Check sheet for the modelled part. Datum: model origin and axes. Units: mm. A direction names the side the tool comes from. Give positions to 0.01 mm unless a question says otherwise; leave off trailing zeros. Order: outer loops, then holes, each group sorted by start corner. A loop starts at its lowest first (then second) coordinate and runs counter-clockwise, first axis right, second up. Notation, with made-up numbers: M -14,78 L 11,78 A30 ccw 11,103 Z; hole C 47.5,-21 d8. An arc over 180 degrees is marked long. Answer in a Markdown table with one row per item. Add a question column.
from build123d import *

# Parameters (mm, degrees)
SKETCH_W           = 180
SKETCH_H           = 180
SKETCH_R           = 2.5
PAD_DEPTH          = 80
SKETCH001_W        = 120
SKETCH001_H        = 80
POCKET_DEPTH       = 11
POCKET002_DEPTH    = 70
POLARPATTERN_COUNT = 4
POCKET003_DEPTH    = 10
SKETCH005_W        = 10
SKETCH005_H        = 30
SKETCH005_H_2      = 25
POCKET004_DEPTH    = 70
SKETCH002_R        = 3
POCKET007_DEPTH    = 11


with BuildPart() as part:
    # Sketch (on Sketch) → Pad (new body)
    with BuildSketch(Plane.XY):
        Rectangle(SKETCH_W, SKETCH_H)
        with Locations((-84, 84)):
            Circle(SKETCH_R, mode=Mode.SUBTRACT)
        with Locations((84, 84)):
            Circle(SKETCH_R, mode=Mode.SUBTRACT)
        with Locations((84, -84)):
            Circle(SKETCH_R, mode=Mode.SUBTRACT)
        with Locations((-84, -84)):
            Circle(SKETCH_R, mode=Mode.SUBTRACT)
        with Locations((-85, 55)):
            Circle(SKETCH_R, mode=Mode.SUBTRACT)
        with Locations((-85, -55)):
            Circle(SKETCH_R, mode=Mode.SUBTRACT)
        with Locations((85, -55)):
            Circle(SKETCH_R, mode=Mode.SUBTRACT)
        with Locations((85, 55)):
            Circle(SKETCH_R, mode=Mode.SUBTRACT)
        with BuildLine():
            Line((-70, 80), (70, 80))
            ThreePointArc((80, 70), (77.071068, 77.071068), (70, 80))
            Line((80, 70), (80, 63.660254))
            ThreePointArc((80, 63.660254), (75, 55), (80, 46.339746))
            Line((80, 46.339746), (80, -46.339746))
            ThreePointArc((80, -46.339746), (75, -55), (80, -63.660254))
            Line((80, -63.660254), (80.000001, -70))
            ThreePointArc((70.000001, -80), (77.071069, -77.071068), (80.000001, -70))
            Line((70.000001, -80), (-69.999999, -80))
            ThreePointArc((-79.999999, -70), (-77.071066, -77.071068), (-69.999999, -80))
            Line((-79.999999, -70), (-79.999999, -63.660253))
            ThreePointArc((-79.999999, -63.660253), (-75, -55), (-79.999999, -46.339747))
            Line((-79.999999, -46.339747), (-79.999999, 46.339747))
            ThreePointArc((-79.999999, 46.339747), (-75, 55), (-79.999999, 63.660253))
            Line((-79.999999, 63.660253), (-79.999999, 69.994765))
            ThreePointArc((-70, 80), (-77.072918, 77.069217), (-79.999999, 69.994765))
        make_face(mode=Mode.SUBTRACT)
    extrude(amount=PAD_DEPTH)

    # Sketch001 (on Face1 of Pad) → Pocket (cut)
    with BuildSketch(Plane(origin=(0, 90, 0), x_dir=(-1, 0, 0), z_dir=(0, 1, 0))):
        with Locations((0, 40)):
            Rectangle(SKETCH001_W, SKETCH001_H)
    extrude(amount=-POCKET_DEPTH, mode=Mode.SUBTRACT)

    # Sketch003 → Pocket002 (cut)
    with BuildSketch(Plane.XY.offset(80)):
        Polygon((-90, 90), (-70, 90), (-90, 70), align=None)
    pocket002 = extrude(amount=-POCKET002_DEPTH, mode=Mode.SUBTRACT)

    # PolarPattern: Pocket002 ×4 about axis
    polarpattern_axis = Axis((0, 0, 80), (0, 0, 1))
    for i in range(1, POLARPATTERN_COUNT):
        add(pocket002.rotate(polarpattern_axis, i * 360 / POLARPATTERN_COUNT), mode=Mode.SUBTRACT)

    # Sketch004 (on Face2 of PolarPattern) → Pocket003 (cut)
    with BuildSketch(Plane(origin=(0, 0, 0), x_dir=(1, 0, 0), z_dir=(0, 0, -1))):
        Polygon((-90, 60), (-83.5, 60), (-80, 57), (-80, 53), (-83.5, 50), (-90, 50), align=None)
        Polygon((83.5, 60), (90, 60), (90, 50), (83.5, 50), (80, 53), (80, 57), align=None)
        Polygon((83.5, -50), (90, -50), (90, -60), (83.5, -60), (80, -57), (80, -53), align=None)
        Polygon((-90, -50), (-83.5, -50), (-80, -53), (-80, -57), (-83.5, -60), (-90, -60), align=None)
    extrude(amount=-POCKET003_DEPTH, mode=Mode.SUBTRACT)

    # Sketch005 (on Face6 of Pocket003) → Pocket004 (cut)
    with BuildSketch(Plane.XY.offset(10)):
        with Locations((-75, 55)):
            Rectangle(SKETCH005_W, SKETCH005_H)
        with Locations((75, 55)):
            Rectangle(SKETCH005_W, SKETCH005_H)
        with Locations((75, -55)):
            Rectangle(SKETCH005_W, SKETCH005_H)
        with Locations((-75, -52.5)):
            Rectangle(SKETCH005_W, SKETCH005_H_2)
    extrude(amount=POCKET004_DEPTH, mode=Mode.SUBTRACT)

    # Sketch002 (on Face30 of Pocket004) → Pocket007 (cut)
    with BuildSketch(Plane(origin=(0, -80, 0), x_dir=(-1, 0, 0), z_dir=(0, 1, 0))):
        with Locations((-50, 5)):
            Circle(SKETCH002_R)
    extrude(amount=-POCKET007_DEPTH, mode=Mode.SUBTRACT)


solid = part.part
Q1. Cross-section at D-D (x = -29). Record the boundary of the cut face in (y, z), and give its area (3 significant figures).
Q2. Go/stop test with flat-tipped pins: pin 1 (8 mm diameter, centred on x = 85, y = 55, fed in from +Z); pin 2 (6.5 mm diameter, centred on x = 84, y = 84, fed in from +Z); pin 3 (6 mm diameter, centred on x = 34, z = 21, fed in from +Y); pin 4 (11 mm diameter, centred on y = 86.5, z = 38.5, fed in from -X). Record where each tip stops, or that it passes through.
Q3. Thickness scan on probe 1 along Y at (x, z) = (-84, 4); probe 2 along X at (y, z) = (84, 5.75); probe 3 along X at (y, z) = (-55, 28). Record the ranges inside material, lowest first.
Q4. Tool access check on faces 1 (the flat face through (82, -82, 10)), 2 (the flat face through (-87, -57, 10)), 3 (the flat face through (87, -57, 10)). Record the directions out of +Z, -Z, +X, -X, +Y, -Y that give a thin tool (end or side, any length) a straight path to the whole face; none if there is none.
Q5. Cross-section at A-A (y = -2). Record the boundary of the cut face in (x, z), and give its area (3 significant figures).
Q6. Cross-section at B-B (x = 50). Record the boundary of the cut face in (y, z), and give its area (3 significant figures).
Q7. Draft check along Y on faces 4 (the cylindrical face through (-86.5, -83.9, 4.9)), 5 (the flat face through (-1, -90, 39)), 6 (the cylindrical face through (76.99, -77.15, 39.44)), 7 (the flat face through (-82, 82, 10)). Enter one of: pulls with the +Y half, pulls with the -Y half, needs draft (parallel to the pull), parting line crosses it, or undercut.
Q8. Cross-section at C-C (z = 49.5). State how many separate pieces and enclosed holes the cut face has, and give its area (3 significant figures).
Values follow:
| question | item | result |
|---|---|---|
| 1 | outline | M -90,0 L -80,0 L -80,80 L -90,80 Z |
| 1 | area | 800 mm² |
| 2 | pin 1 | z = 80 |
| 2 | pin 2 | z = 10 |
| 2 | pin 3 | y = -80 |
| 2 | pin 4 | x = -79 |
| 3 | probe 1 | -90 to -86.5, -81.5 to -60, -50 to 50, 60 to 81.5, 86.5 to 90 |
| 3 | probe 2 | -90 to -86.5, -81.5 to -60, 60 to 81.5, 86.5 to 90 |
| 3 | probe 3 | -90 to -87.5, -82.5 to -80, 80 to 82.5, 87.5 to 90 |
| 4 | face 1 | +Z, +X, -Y |
| 4 | face 2 | -Z, -X |
| 4 | face 3 | -Z, +X |
| 5 | outline | M -90,0 L -80,0 L -80,80 L -90,80 Z; M 80,0 L 90,0 L 90,80 L 80,80 Z |
| 5 | area | 1,600 mm² |
| 6 | outline | M -90,0 L -80,0 L -80,2 L -90,2 Z; M -90,8 L -80,8 L -80,80 L -90,80 Z |
| 6 | area | 740 mm² |
| 7 | face 4 | undercut |
| 7 | face 5 | pulls with the -Y half |
| 7 | face 6 | undercut |
| 7 | face 7 | needs draft |
| 8 | separate pieces | 1 |
| 8 | enclosed holes | 4 |
| 8 | area | 4,810 mm² |
